Here's how the part is built. I have some questions about the finished solid (model axes, mm). Face numbers are marked on the shaded views. Give positions to 0.01 mm unless a question says otherwise; leave off trailing zeros. Write each loop counter-clockwise with the first axis right and the second up, starting at its lowest first coordinate (ties: lowest second). Pieces come first, ordered by that corner, then holes. Notation, with made-up numbers: (33, -26) - (77, -26) arc R33 cw to (77, 11) - close; hole circle Ø8 at (46, 41). An arc over 180 degrees is marked (long way). One line per item, written item: value. Start each with the question number.
1) Imagine slicing it at C-C on y = -31. Write out the boundary of the cut face in (x, z), plus the area to 3 significant figures.
2) We'd pull the mould along Z, two halves only. Please class the marked faces 1, 2 and 3: +Z half, -Z half, draft (parallel to the pull), parting line (faces both ways), or undercut.
3) I'm going to push flat-ended pins straight in: P1, Ø10, axis at x = -134.5, z = -11.5, coming from the -Y side; P2, Ø3.5, axis at x = -118.5, z = 5, coming from the -Y side; P3, Ø5, axis at x = -141, z = 15, coming from the -Y side. Where does each tip first touch, or does it pass through?
4) Please list where these lines run through material, in increasing order: L1, parallel to Z at x = -158, y = -7.5; L2, parallel to X at y = 3, z = 10.5; L3, parallel to X at y = -16, z = -13. Write a range as [from, to].
5) Imagine slicing it at B-B on y = -3.5. Write out the boundary of the cut face in (x, z).
6) Imagine slicing it at D-D on z = 14. Write out the boundary of the cut face in (x, y), plus the area to 3 significant figures.
7) Imagine slicing it at A-A on x = -135. Write out the boundary of the cut face in (y, z), plus the area to 3 significant figures.
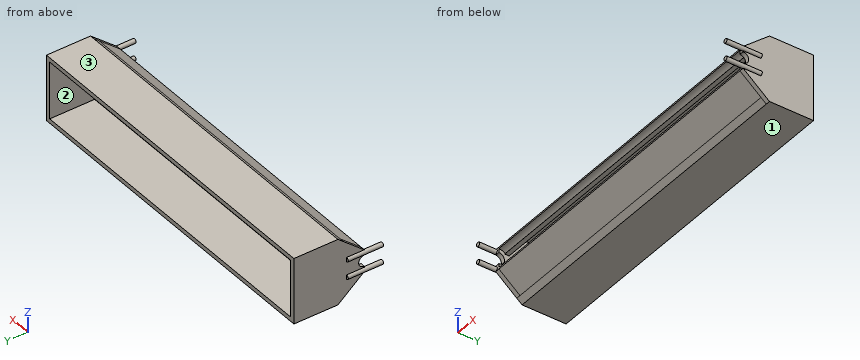
from build123d import *

# Parameters (mm, degrees)
BOSS_EXTRUDE1_DEPTH      = 2.54
BOSS_EXTRUDE2_DEPTH      = 196.342
CUT_EXTRUDE2_DEPTH       = 200.22892422
CUT_EXTRUDE2_DEPTH_BACK  = 200.22892422
SKETCH6_R                = 3.2385
SKETCH9_R                = 1.261392003
BOSS_EXTRUDE5_DEPTH      = 10.16
MIRROR11_COPY_1_SKETCH_R = 1.261392003
MIRROR11_COPY_1_DEPTH    = 10.16
BOSS_EXTRUDE6_DEPTH      = 191.262


with BuildPart() as part:
    # Sketch2 → Boss-Extrude1 (new body)
    with BuildSketch(Plane(origin=(0, 0, 0), x_dir=(0, 0, -1), z_dir=(1, 0, 0))):
        Polygon((-19.05, -12.7), (-6.35, -27.912018594), (6.35, -27.912018594), (19.05, -12.7), (19.05, 12.7), (-19.05, 12.7), align=None)
    boss_extrude1 = extrude(amount=BOSS_EXTRUDE1_DEPTH)

    # Sketch3 → Boss-Extrude2 (add)
    with BuildSketch(Plane(origin=(2.54, 0, 0), x_dir=(0, 0, -1), z_dir=(1, 0, 0))):
        Polygon((16.51, -13.202403719), (16.51, 12.7), (19.05, 12.7), (19.05, -12.7), (16.51, -15.742403719), (3.81, -24.559218594), (3.81, -22.019218594), align=None)
    boss_extrude2 = extrude(amount=-BOSS_EXTRUDE2_DEPTH)

    # Mirror1: Boss-Extrude2 across plane
    add(boss_extrude2.mirror(Plane.XY))

    # Mirror3: Boss-Extrude1 across plane
    add(boss_extrude1.mirror(Plane(origin=(-95.631, 0, 0), x_dir=(0, 0, 1), z_dir=(1, 0, 0))))

    # Sketch6 → Cut-Extrude2 (cut, two sides: drawn at the far end of the back side and taken through both)
    with BuildSketch(Plane.ZY.offset(193.802).offset(-CUT_EXTRUDE2_DEPTH_BACK)):
        with Locations((0, -27.912018594)):
            Circle(SKETCH6_R)
    extrude(amount=CUT_EXTRUDE2_DEPTH + CUT_EXTRUDE2_DEPTH_BACK, mode=Mode.SUBTRACT)

    # Sketch9 → Boss-Extrude5 (add, symmetric)
    with BuildSketch(Plane.XZ.offset(27.912018594)):
        with Locations(Location((2.54, 5.088607997, 0), (0, 0, 270))):
            Circle(SKETCH9_R)
    boss_extrude5 = extrude(amount=BOSS_EXTRUDE5_DEPTH, both=True)

    # Mirror10: Boss-Extrude5 across plane
    add(boss_extrude5.mirror(Plane(origin=(-95.631, 0, 0), x_dir=(0, 0, 1), z_dir=(1, 0, 0))))

    # Mirror11: Boss-Extrude5 across plane
    add(boss_extrude5.mirror(Plane.XY))

    # Mirror11 copy 1 sketch → Mirror11 copy 1 (add, symmetric)
    with BuildSketch(Plane(origin=(-191.262, -27.912018594, 0), x_dir=(-1, 0, 0), z_dir=(0, -1, 0))):
        with Locations(Location((2.54, 5.088607997, 0), (0, 0, 270))):
            Circle(MIRROR11_COPY_1_SKETCH_R)
    extrude(amount=MIRROR11_COPY_1_DEPTH, both=True)

    # Sketch10 → Boss-Extrude6 (add)
    with BuildSketch(Plane.ZY):
        with BuildLine():
            Line((-4.128889044, -24.337833896), (-16.51, -15.742403719))
            Line((-16.51, -15.742403719), (-6.35, -27.912018594))
            Line((-6.35, -27.912018594), (-5.461, -27.912018594))
            ThreePointArc((-5.461, -27.912018594), (-5.117146865, -26.004840322), (-4.128889044, -24.337833896))
        make_face()
    boss_extrude6 = extrude(amount=BOSS_EXTRUDE6_DEPTH)

    # Mirror12: Boss-Extrude6 across plane
    add(boss_extrude6.mirror(Plane.XY))


solid = part.part
Numbers:
1. outline: circle Ø2.52 at (-193.8, -5.09); circle Ø2.52 at (-193.8, 5.09); circle Ø2.52 at (2.54, -5.09); circle Ø2.52 at (2.54, 5.09)
1. area: 20.0 mm^2
2. face 1: -Z half
2. face 2: undercut
2. face 3: +Z half
3. P1: y = -27.73
3. P2: y = -27.91
3. P3: y = -20.55
4. L1: [-19.05, -16.51], [16.51, 19.05]
4. L2: [-193.8, -191.26], [0, 2.54]
4. L3: [-193.8, 2.54]
5. outline: (-193.8, -19.05) - (2.54, -19.05) - (2.54, 19.05) - (-193.8, 19.05) - close; hole (-191.26, -16.51) - (0, -16.51) - (0, 16.51) - (-191.26, 16.51) - close
6. outline: (-193.8, -18.75) - (2.54, -18.75) - (2.54, 12.7) - (0, 12.7) - (0, -14.94) - (-191.26, -14.94) - (-191.26, 12.7) - (-193.8, 12.7) - close
6. area: 887 mm^2
7. outline: (-27.91, -6.35) - (-12.7, -19.05) - (12.7, -19.05) - (12.7, -16.51) - (-13.2, -16.51) - (-22.02, -3.81) - (-24.56, -3.81) - (-24.34, -4.13) arc R5.46 cw to (-27.91, -5.46) - close; (-27.91, 5.46) arc R5.46 cw to (-24.34, 4.13) - (-24.56, 3.81) - (-22.02, 3.81) - (-13.2, 16.51) - (12.7, 16.51) - (12.7, 19.05) - (-12.7, 19.05) - (-27.91, 6.35) - close
7. area: 266 mm^2
